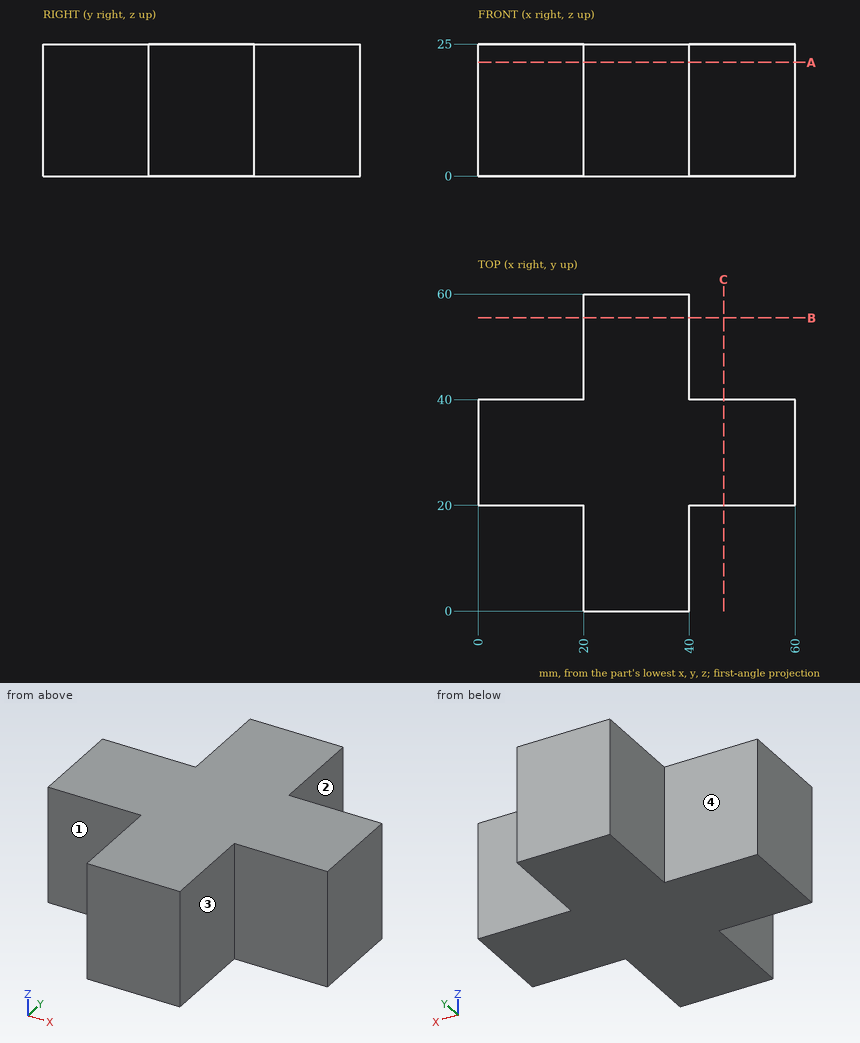
Design review of the part shown in the three views and the two pictorial views. Dimensions are in mm from the part's minimum x, y and z. A direction names the side the tool comes from. Coordinates: 2 decimals unless noted, no trailing zeros. Order: outer loops, then holes, each group sorted by start corner. A loop starts at its lowest first (then second) coordinate and runs counter-clockwise, first axis right, second up. Notation, with made-up numbers: (39.5, 11.5) -> (77.5, 11.5) arc R19 cw to (77.5, 30.5) -> close; hole circle Ø10 at (5.25, 63.5). An arc over 180 degrees is marked (long way). Use one line per item in the form item = value. Start each with the question number.
(1) Add section A-A on z = 21.5. State the section outline as (x, y) points, plus the area to 3 significant figures.
(2) For probe 1 along Y at (x, z) = (10, 7.75), list the stretches that pass through material, from the lowest coordinate up.
(3) For the marked faces 1, 2, 3 and 4, list the 3-axis set-ups (+Z, -Z, +X, -X, +Y, -Y) from which the entire face can be reached by the end or side of a thin tool; tool diameter is ignored.
(4) Insertion check: pin 1 (10 mm diameter, centred on y = 52, z = 8.5, fed in from -X); pin 2 (10 mm diameter, centred on y = 6, z = 17.5, fed in from +X); pin 3 (1 mm diameter, centred on x = 14.5, z = 22.5, fed in from +Y). Each pin has a flat end and moves straight along its axis. Give the tip position at first contact, or say it passes through.
(5) Add section B-B on y = 55.5. State the section outline as (x, z) points, plus the area to 3 significant figures.
Answer block:
q1.outline = (0, 20) -> (20, 20) -> (20, 0) -> (40, 0) -> (40, 20) -> (60, 20) -> (60, 40) -> (40, 40) -> (40, 60) -> (20, 60) -> (20, 40) -> (0, 40) -> close
q1.area = 2,000 mm²
q2.probe_1 = 20 to 40
q3.face_1 = +Z, -Z, -X, -Y
q3.face_2 = +Z, -Z, +X, +Y
q3.face_3 = +Z, -Z, +X, -Y
q3.face_4 = +Z, -Z, -X, +Y
q4.pin_1 = 20
q4.pin_2 = 40
q4.pin_3 = 40
q5.outline = (20, 0) -> (40, 0) -> (40, 25) -> (20, 25) -> close
q5.area = 500 mm²
